Here's how the part is built. I have some questions about the finished solid (model axes, mm). A direction names the side the tool comes from. Coordinates: 2 decimals unless noted, no trailing zeros. Write each loop counter-clockwise with the first axis right and the second up, starting at its lowest first coordinate (ties: lowest second). Pieces come first, ordered by that corner, then holes.
(1) Thinking about a two-plate mould opening in Z: for faces 3 (the flat face through (0, 0, 5)), 4 (the flat face through (3.5, -2, 2)), which applies, released by +Z, released by -Z, zero draft, split by the parting line, or undercut?
(2) Imagine slicing it at D-D, the plane z = 0.25. List the corners of the cut face in (x, y) for me, plus the area to 3 significant figures.
(3) For pin 1 Ø0.9 at (x, z) = (1, 1.5) entering from -Y; pin 2 Ø3 at (y, z) = (-0.5, -3) entering from +X; pin 3 Ø1.6 at (x, z) = (0, 3.5) entering from -Y, each with a flat end and sliding along its axis, tell me the tip position at first contact or that it passes through.
(4) Imagine slicing it at C-C, the plane y = -4.25. List the corners of the cut face in (x, z) for me, plus the area to 3 significant figures.
(5) Imagine slicing it at A-A, the plane z = 2.75. List the corners of the cut face in (x, y) for me, plus the area to 3 significant figures.
(6) Please list where these lines run through material, in increasing order: probe 1 along Y at (x, z) = (0, 3.15); probe 2 along Y at (x, z) = (-1, 1.75); probe 3 along Z at (x, y) = (2.5, -3).
(7) Which directions (+Z, -Z, +X, -X, +Y, -Y) give clear straight access to the entire face, cutting with the end or side of a thin tool? Please do faces 1 (the cylindrical face through (-0.1, 3.5, 2.2)), 2 (the cylindrical face through (-3, 0, 3)).
```python
from build123d import *

# Parameters (mm, degrees)
EXTRUDE_2_DEPTH     = 4.5
SKETCH_2_R          = 3
CUT_EXTRUDE_1_DEPTH = 3.5
SKETCH_3_R          = 2.8
EXTRUDE_3_DEPTH     = 4
CUT_EXTRUDE_2_DEPTH = 1.5
SWEEP_2_PROFILE_R   = 0.35
SWEEP_3_PROFILE_R   = 0.35
FILLET_1_R          = 1


with BuildPart() as part:
    # Эскиз1 → Бобышка-Вытянуть2 (new body)
    with BuildSketch(Plane.XY):
        with BuildLine():
            Line((-3.5, -3.5), (-3.5, 0))
            ThreePointArc((-3.5, 0), (0, 3.5), (3.5, 0))
            Line((3.5, 0), (3.5, -3.5))
            Line((3.5, -3.5), (3.5, -5))
            Line((3.5, -5), (-3.5, -5))
            Line((-3.5, -5), (-3.5, -3.5))
        make_face()
    extrude(amount=EXTRUDE_2_DEPTH)

    # Эскиз2 → Вырез-Вытянуть1 (cut)
    with BuildSketch(Plane.XY.offset(4.5)):
        Circle(SKETCH_2_R)
    extrude(amount=-CUT_EXTRUDE_1_DEPTH, mode=Mode.SUBTRACT)

    # Эскиз3 → Бобышка-Вытянуть3 (add)
    with BuildSketch(Plane.XY.offset(1)):
        Circle(SKETCH_3_R)
    extrude(amount=EXTRUDE_3_DEPTH)

    # Эскиз4 → Вырез-Вытянуть2 (cut)
    with BuildSketch(Plane.XZ.offset(5)):
        Polygon((0.146156233, 3), (-3.5, 3), (-3.5, 0), (3.5, 0), (3.5, 3), align=None)
    extrude(amount=-CUT_EXTRUDE_2_DEPTH, mode=Mode.SUBTRACT)

    # По траектории2: sweep along a path in Эскиз6
    with BuildLine(Plane.ZY) as sweep_2_path:
        Line((0, -1.27), (-1.5, -1.27))
        ThreePointArc((-1.5, -1.27), (-2.207106781, -1.562893219), (-2.5, -2.27))
        Line((-2.5, -2.27), (-2.5, -5))
        Line((-2.5, -5), (-2.5, -7))
    # По траектории2 profile (on start of the path) → По траектории2 (sweep)
    with BuildSketch(Plane(origin=(0, -1.27, 0), x_dir=(-1, 0, 0), z_dir=(0, 0, -1))):
        Circle(SWEEP_2_PROFILE_R)
    sweep(path=sweep_2_path.line)

    # По траектории3: sweep along a path in Эскиз107
    with BuildLine(Plane.ZY) as sweep_3_path:
        Line((0, 1.27), (-3, 1.27))
        ThreePointArc((-3, 1.27), (-4.414213562, 0.684213562), (-5, -0.73))
        Line((-5, -0.73), (-5, -6.984666466))
    # По траектории3 profile (on start of the path) → По траектории3 (sweep)
    with BuildSketch(Plane(origin=(0, 1.27, 0), x_dir=(0, -1, 0), z_dir=(0, 0, -1))):
        Circle(SWEEP_3_PROFILE_R)
    sweep(path=sweep_3_path.line)

    # Скругление1
    fillet_1_edges = [part.edges().sort_by_distance(p)[0] for p in [
        (-2.8, 0, 5),
    ]]
    fillet(fillet_1_edges, radius=FILLET_1_R)


solid = part.part
```
Recorded:
1. face 3: released by +Z
1. face 4: zero draft
2. outline: (-3.5, -3.5) - (3.5, -3.5) - (3.5, 0) arc R3.5 ccw to (-3.5, 0) - close
2. area: 43.7 mm2
3. pin 1: stops at y = -3.5
3. pin 2: stops at x = 0.35
3. pin 3: stops at y = -5
4. outline: (-3.5, 3) - (3.5, 3) - (3.5, 4.5) - (-3.5, 4.5) - close; circle Ø0.7 at (0, -5); circle Ø0.7 at (0, -2.5)
4. area: 11.3 mm2
5. outline: (-3.5, -3.5) - (3.5, -3.5) - (3.5, 0) arc R3.5 ccw to (-3.5, 0) - close; circle Ø5.6 at (0, 0); hole circle Ø6 at (0, 0)
5. area: 40.1 mm2
6. probe 1: y = -5 to -3, -2.8 to 2.8, 3 to 3.5
6. probe 2: y = -3.5 to -2.83, -2.62 to 2.62, 2.83 to 3.35
6. probe 3: z = 0 to 4.5
7. face 1: +Z, -Z, +Y
7. face 2: +Z
